Verification items for this drawing (mm, ordinates from the low corner). A direction names the side the tool comes from. Round coordinates to 2 decimals unless told otherwise and drop trailing zeros. Loops run counter-clockwise (first coordinate to the right, second up) from the corner with the lowest first, then second, coordinate; pieces in that order, holes last. Notation, with made-up numbers: (20.25, 69.5) - (32.25, 69.5) arc R22 ccw to (32.25, 78.5) - close; hole circle Ø5 at (-26, 69). An arc over 180 degrees is marked (long way). Use a Markdown table: item, result. Add a question column.
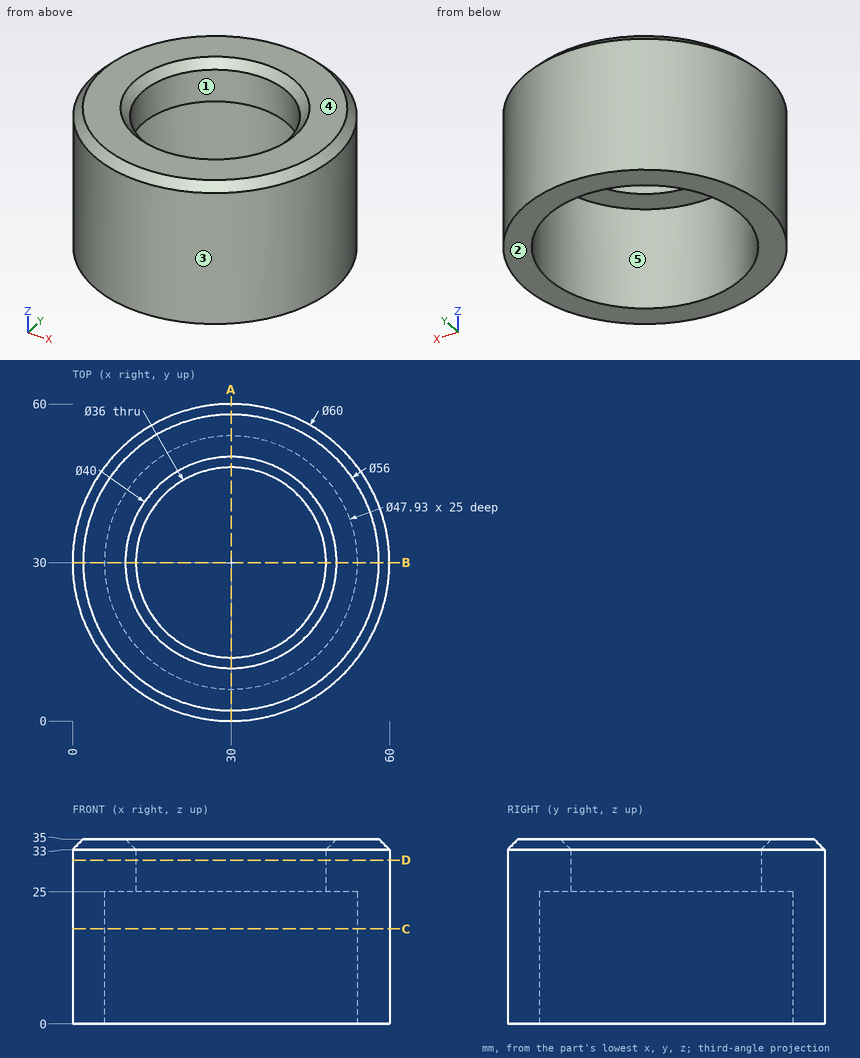
Q1. Section check D-D on z = 31. Record the cut outline in (x, y).
Q2. Release check for a two-part mould opening along Y. For the marked faces 1, 2 and 3 record: +Y half, -Y half, draft (parallel to the pull), parting line (faces both ways), or undercut.
Q3. Section check A-A on x = 30. Record the cut outline in (y, z) (3 decimals).
Q4. Section check C-C on z = 18. Record the cut outline in (x, y) (3 decimals).
Q5. Thickness scan on line 1 along Y through (x, z) = (30, 28.5); line 2 along Y through (x, z) = (30, 6.5) (3 decimals); line 3 along Z through (x, y) = (11.5, 16.5). Record the ranges inside material, lowest first.
Q6. Set-up check for the marked faces 4 and 5: record each of +Z, -Z, +X, -X, +Y, -Y from which the full face is reachable in a straight line by a thin tool's end or side.
Q7. Go/stop test with flat-tipped pins: pin 1 Ø2 at (x, z) = (49, 4) entering from -Y; pin 2 Ø1 at (y, z) = (35.5, 14) entering from +X; pin 3 Ø4 at (x, z) = (40.5, 7) entering from +Y. Record where each tip stops, or that it passes through.
Determined:
| question | item | result |
|---|---|---|
| 1 | outline | circle Ø60 at (30, 30); hole circle Ø36 at (30, 30) |
| 2 | face 1 | undercut |
| 2 | face 2 | draft |
| 2 | face 3 | parting line |
| 3 | outline | (0, 0) - (6.035, 0) - (6.035, 25) - (12, 25) - (12, 33) - (10, 35) - (2, 35) - (0, 33) - close; (48, 25) - (53.965, 25) - (53.965, 0) - (60, 0) - (60, 33) - (58, 35) - (50, 35) - (48, 33) - close |
| 4 | outline | circle Ø60 at (30, 30); hole circle Ø47.93 at (30, 30) |
| 5 | line 1 | y = 0 to 12, 48 to 60 |
| 5 | line 2 | y = 0 to 6.035, 53.965 to 60 |
| 5 | line 3 | z = 25 to 35 |
| 6 | face 4 | +Z, +X, -X, +Y, -Y |
| 6 | face 5 | -Z |
| 7 | pin 1 | stops at y = 6 |
| 7 | pin 2 | stops at x = 59.58 |
| 7 | pin 3 | stops at y = 58.77 |
